from build123d import *

# Parameters (mm, degrees)
EXTRUDE_1_DEPTH     = 20
SKETCH_2_R          = 5.65
CUT_EXTRUDE_1_DEPTH = 5.5
CUT_EXTRUDE_START   = -6
CUT_EXTRUDE_4_DEPTH = 8
EXTRUDE_START       = 5
SKETCH_5_R          = 1.5
EXTRUDE_2_DEPTH     = 3
CUT_EXTRUDE_5_REACH = 149.085
SKETCH_7_R          = 3
EXTRUDE_3_DEPTH     = 6
EXTRUDE_4_DEPTH     = 8
EXTRUDE_5_DEPTH     = 8
EXTRUDE_6_DEPTH     = 6
SKETCH_12_R         = 2
CUT_EXTRUDE_7_DEPTH = 14


with BuildPart() as part:
    # 草图1 → 凸台-拉伸1 (new body)
    with BuildSketch(Plane.XY):
        with BuildLine():
            Line((35.26398638, -8), (88.563757686, -105.288040462))
            ThreePointArc((88.563757686, -105.288040462), (95.239080336, -107.332125442), (97.455297675, -100.711959538))
            Line((97.455297675, -100.711959538), (47.113231991, 3.660864739))
            ThreePointArc((47.113231991, 3.660864739), (44.166118222, 6.829601669), (40, 8))
            Line((40, 8), (6, 8))
            ThreePointArc((6, 8), (-10, 0), (6, -8))
            Line((6, -8), (35.26398638, -8))
        make_face()
    extrude(amount=EXTRUDE_1_DEPTH)

    # 草图2 → 切除-拉伸1 (cut)
    with BuildSketch(Plane.XY.offset(20)):
        Circle(SKETCH_2_R)
    extrude(amount=-CUT_EXTRUDE_1_DEPTH, mode=Mode.SUBTRACT)

    # 草图4 → 切除-拉伸4 (cut)
    with BuildSketch(Plane(origin=(0, 0, 0), x_dir=(-1, 0, 0), z_dir=(0, 0, -1)).offset(CUT_EXTRUDE_START)):
        with BuildLine():
            Line((-97.455297675, -100.711959538), (-93.978649208, -93.503919609))
            Line((-93.978649208, -93.503919609), (-84.718676675, -98.269616408))
            Line((-84.718676675, -98.269616408), (-88.563757686, -105.288040462))
            ThreePointArc((-88.563757686, -105.288040462), (-95.297568142, -107.445769995), (-97.455297675, -100.711959538))
        make_face()
    extrude(amount=-CUT_EXTRUDE_4_DEPTH, mode=Mode.SUBTRACT)

    # 草图5 → 凸台-拉伸2 (add)
    with BuildSketch(Plane.XY.offset(6).offset(EXTRUDE_START)):
        with Locations((92.950272719, -102.88486483)):
            Circle(SKETCH_5_R)
    extrude(amount=EXTRUDE_2_DEPTH)

    # 草图7 → 切除-拉伸5 (cut, up to next)
    with BuildSketch(Plane(origin=(0, 0, 0), x_dir=(-1, 0, 0), z_dir=(0, 0, -1)), mode=Mode.PRIVATE) as cut_extrude_5_sk1:
        with Locations((-92.950272719, -102.88486483)):
            Circle(SKETCH_7_R)
    cut_extrude_5_tool1 = extrude(cut_extrude_5_sk1.sketch, amount=-CUT_EXTRUDE_5_REACH, mode=Mode.PRIVATE) & part.part
    add(cut_extrude_5_tool1.solids().sort_by_distance((92.950273, -102.884865, 0))[0], mode=Mode.SUBTRACT)

    # 草图8 → 凸台-拉伸3 (add)
    with BuildSketch(Plane(origin=(0, 0, 0), x_dir=(-1, 0, 0), z_dir=(0, 0, -1))):
        with BuildLine():
            Line((-95.617734716, -101.512040553), (-101.841812708, -98.308783906))
            Line((-101.841812708, -98.308783906), (-109.392346233, -112.979824888))
            Line((-109.392346233, -112.979824888), (-91.609266255, -122.131986736))
            Line((-91.609266255, -122.131986736), (-84.05873273, -107.460945754))
            Line((-84.05873273, -107.460945754), (-90.282810723, -104.257689107))
            ThreePointArc((-90.282810723, -104.257689107), (-94.323096996, -105.552326827), (-95.617734716, -101.512040553))
        make_face()
    extrude(amount=-EXTRUDE_3_DEPTH)

    # 草图9 → 凸台-拉伸4 (add)
    with BuildSketch(Plane(origin=(0, 0, 0), x_dir=(-1, 0, 0), z_dir=(0, 0, -1))):
        Polygon((-106.417893632, -107.200323895), (-88.634813654, -116.352485743), (-91.609266255, -122.131986736), (-109.392346233, -112.979824888), align=None)
    extrude(amount=EXTRUDE_4_DEPTH)

    # 草图10 → 凸台-拉伸5 (add)
    with BuildSketch(Plane(origin=(0, 0, 0), x_dir=(-1, 0, 0), z_dir=(0, 0, -1))):
        Polygon((-88.113569936, -71.634163939), (-70.330489958, -80.786325787), (-67.356037358, -75.006824794), (-85.139117336, -65.854662946), align=None)
    extrude(amount=EXTRUDE_5_DEPTH)

    # 草图11 → 凸台-拉伸6 (add)
    with BuildSketch(Plane.XY):
        Polygon((81.536815817, -67.708607626), (84.361592697, -73.565140068), (88.113569936, -71.634163939), (85.139117336, -65.854662946), align=None)
        Polygon((67.356037358, -75.006824794), (70.330489958, -80.786325787), (74.082467198, -78.855349657), (70.958338877, -73.152880114), align=None)
    extrude(amount=EXTRUDE_6_DEPTH)

    # 草图12 → 切除-拉伸7 (cut)
    with BuildSketch(Plane(origin=(0, 0, -8), x_dir=(-1, 0, 0), z_dir=(0, 0, -1))):
        with Locations((-103.459349938, -112.378114854)):
            Circle(SKETCH_12_R)
        with Locations((-94.567809949, -116.954195778)):
            Circle(SKETCH_12_R)
        with Locations((-73.289033653, -75.608534828)):
            Circle(SKETCH_12_R)
        with Locations(Location((-82.180573642, -71.032453904, 0), (0, 0, 89.850321616))):
            Circle(SKETCH_12_R)
    extrude(amount=-CUT_EXTRUDE_7_DEPTH, mode=Mode.SUBTRACT)


solid = part.part
The listing builds one solid part. Answer for the finished solid, in the listing's coordinates (mm). A direction names the side the tool comes from. Round coordinates to 2 decimals unless told otherwise and drop trailing zeros. Write each loop counter-clockwise with the first axis right and the second up, starting at its lowest first coordinate (ties: lowest second). Pieces come first, ordered by that corner, then holes. Notation, with made-up numbers: (82, 88) - (141, 88) arc R33 ccw to (141, 116) - close; hole circle Ø9 at (-8, 12.25). An arc over 180 degrees is marked (long way). Use one line per item in the form item = value. Start each with the question number.
Item 1: A tool of negligible diameter and unlimited length cuts with its end or side. For faces 1 (the flat face through (71, -77, 6)), 2 (the flat face through (93, -101, 14)), 3 (the flat face through (23, 8, 10)), from which of +Z, -Z, +X, -X, +Y, -Y can it reach the whole face along a straight path? Write none if from no direction.
Item 2: Find the intervals of material crossed by line 1 (Y direction, x = 26.5, z = 1.5); line 2 (X direction, y = -79.5, z = 3); line 3 (Z direction, x = 92, y = -101), in increasing order. Write a range as [from, to].
Item 3: A cutting plane is placed at C-C (z = -4). Write down the section's boundary in (x, y).
Item 4: A cutting plane is placed at B-B (x = 0). Write down the section's boundary in (y, z).
Item 5: A cutting plane is placed at D-D (y = 0). Write down the section's boundary in (x, z).
Item 6: Flat-ended cylindrical pins translate along their axes: pin 1 Ø1.5 at (x, y) = (92.5, -102.5) entering from -Z; pin 2 Ø2.5 at (x, y) = (94.57, -116.95) entering from +Z; pin 3 Ø12 at (y, z) = (-11, 6.5) entering from +X; pin 4 Ø3 at (x, y) = (82.18, -71.03) entering from -Z. Find the tip coordinate at first contact, or state that the pin passes through.
Item 7: A cutting plane is placed at A-A (z = 16.75). Write down the section's boundary in (x, y), plus the area to 3 significant figures.
Item 8: Determine the mould class of faces 4 (the flat face through (0, 0, 14.5)), 5 (the flat face through (61.54, -55.96, 9.86)), 6 (the flat face through (89.413, -95.853, 9.944)) for opening direction Z: +Z half, -Z half, draft (parallel to the pull), parting line (faces both ways), or undercut.
The answers:
q1.face_1 = +Z, -X, -Y
q1.face_2 = none
q1.face_3 = +Z, -Z, +X, +Y
q2.line_1 = [-8, 8]
q2.line_2 = [69.67, 72.83], [74.44, 87.22]
q2.line_3 = [14, 20]
q3.outline = (67.36, -75.01) - (70.33, -80.79) - (88.11, -71.63) - (85.14, -65.85) - close; (88.63, -116.35) - (91.61, -122.13) - (109.39, -112.98) - (106.42, -107.2) - close; hole circle Ø4 at (73.29, -75.61); hole circle Ø4 at (82.18, -71.03); hole circle Ø4 at (94.57, -116.95); hole circle Ø4 at (103.46, -112.38)
q4.outline = (-10, 0) - (10, 0) - (10, 20) - (5.65, 20) - (5.65, 14.5) - (-5.65, 14.5) - (-5.65, 20) - (-10, 20) - close
q5.outline = (-10, 0) - (48.88, 0) - (48.88, 20) - (5.65, 20) - (5.65, 14.5) - (-5.65, 14.5) - (-5.65, 20) - (-10, 20) - close
q6.pin_1 = 11
q6.pin_2 = through
q6.pin_3 = 57.08
q6.pin_4 = 6
q7.outline = (6, -8) - (35.26, -8) - (88.56, -105.29) arc R5 ccw to (97.46, -100.71) - (47.11, 3.66) arc R8 ccw to (40, 8) - (6, 8) arc R10 ccw (long way) to start; hole circle Ø11.3 at (0, 0)
q7.area = 2,250 mm^2
q8.face_4 = +Z half
q8.face_5 = draft
q8.face_6 = undercut
